from build123d import *

# Parameters (mm, degrees)
BASPROSKE_W                                    = 5
BASPROSKE_H                                    = 22
TOOTHCUT_DEPTH                                 = 32.511902513
TEETHCUTS_COUNT                                = 20
TEETHCUTS_ANGLE                                = 342
BORSKE_R                                       = 3.5
BORE_DEPTH                                     = 50.0000508
FRAISAGE_POUR_VIS_T_TE_FRAIS_E_M21_D           = 2.4
FRAISAGE_POUR_VIS_T_TE_FRAIS_E_M21_CSINK_D     = 4.4
FRAISAGE_POUR_VIS_T_TE_FRAIS_E_M21_CSINK_ANGLE = 90
R_P_TITION_CIRCULAIRE1_COUNT                   = 4


with BuildPart() as part:
    # BasProSke → Base-Revolve (revolve)
    with BuildSketch(Plane(origin=(0, 0, 0), x_dir=(1, 0, 0), z_dir=(0, 1, 0)), mode=Mode.PRIVATE) as base_revolve_sk:
        with Locations((2.5, 11)):
            Rectangle(BASPROSKE_W, BASPROSKE_H)
    revolve(base_revolve_sk.sketch.rotate(Axis((-10, 0, 0), (1, 0, 0)), 180), axis=Axis((-10, 0, 0), (1, 0, 0)))

    # TooCutSke → ToothCut (cut, through all)
    with BuildSketch(Plane(origin=(0, 0, 0), x_dir=(0, 0, -1), z_dir=(1, 0, 0))):
        with BuildLine():
            ThreePointArc((0.986171591, 17.471189616), (0, 17.499), (-0.986171591, 17.471189616))
            ThreePointArc((-0.986171591, 17.471189616), (-1.626916196, 19.798789858), (-2.932850173, 21.829260982))
            ThreePointArc((-2.932850173, 21.829260982), (0, 22.0254), (2.932850173, 21.829260982))
            ThreePointArc((2.932850173, 21.829260982), (1.626916196, 19.798789858), (0.986171591, 17.471189616))
        make_face()
    toothcut = extrude(amount=TOOTHCUT_DEPTH, mode=Mode.SUBTRACT)

    # TeethCuts: ToothCut ×20 about axis
    teethcuts_axis = Axis((-10, 0, 0), (1, 0, 0))
    for i in range(1, TEETHCUTS_COUNT):
        add(toothcut.rotate(teethcuts_axis, i * TEETHCUTS_ANGLE / (TEETHCUTS_COUNT - 1)), mode=Mode.SUBTRACT)

    # BorSke → Bore (cut, symmetric)
    with BuildSketch(Plane(origin=(0, 0, 0), x_dir=(0, 0, -1), z_dir=(1, 0, 0))):
        with Locations(Location((0, 0, 0), (0, 0, 180))):
            Circle(BORSKE_R)
    extrude(amount=BORE_DEPTH, both=True, mode=Mode.SUBTRACT)

    # Fraisage pour vis à tête fraisée M21 (through all)
    with Locations(Plane.ZY):
        with Locations((0, 8)):
            fraisage_pour_vis_t_te_frais_e_m21 = CounterSinkHole(FRAISAGE_POUR_VIS_T_TE_FRAIS_E_M21_D / 2, FRAISAGE_POUR_VIS_T_TE_FRAIS_E_M21_CSINK_D / 2, counter_sink_angle=FRAISAGE_POUR_VIS_T_TE_FRAIS_E_M21_CSINK_ANGLE)

    # Répétition circulaire1: Fraisage pour vis à tête fraisée M21 ×4 about axis
    r_p_tition_circulaire1_axis = Axis((0, 0, 0), (1, 0, 0))
    for i in range(1, R_P_TITION_CIRCULAIRE1_COUNT):
        add(fraisage_pour_vis_t_te_frais_e_m21.rotate(r_p_tition_circulaire1_axis, i * 360 / R_P_TITION_CIRCULAIRE1_COUNT), mode=Mode.SUBTRACT)


solid = part.part
Design review of the part built by this model. Coordinates are the model's own, in mm. A direction names the side the tool comes from. Coordinates: 2 decimals unless noted, no trailing zeros. Write each loop counter-clockwise with the first axis right and the second up, starting at its lowest first coordinate (ties: lowest second). Pieces come first, ordered by that corner, then holes. Notation, with made-up numbers: (87.5, 36) -> (146.5, 36) arc R7 cw to (146.5, 44) -> close; hole circle Ø3 at (85.5, -32). An arc over 180 degrees is marked (long way). Write each question's results on one line, items separated by ' | '. Start each with the question number.
(1) For line 1 along Y through (x, z) = (0.7, -19); line 2 along Y through (x, z) = (4.4, 15.5); line 3 along Z through (x, y) = (2.75, 0.5), list the stretches that pass through material, from the lowest coordinate up. Write a range as from..to.
(2) Tool access review of faces 1 (the face through (2.465, 19.754, 1.607)), 2 (the face through (2.465, -15.037, -12.911)), 3 (the face through (2.46, 14.17, 10.27)): name each direction out of +Z, -Z, +X, -X, +Y, -Y from which nothing blocks a thin tool from reaching the whole face with its end or side.
(3) Clearance check with flat-ended pins moving along their axes: P1, Ø1.5, axis at x = 0.5, y = 4, coming from the +Z side; P2, Ø3, axis at x = 1.5, z = -12.5, coming from the -Y side. State where each tip first meets the part, or that it passes through.
(4) The part is to be moulded in two halves that separate along Z. For faces 4 (the face through (2.46, -7.63, 18.29)), 5 (the face through (2.46, -16.64, 5.42)), 6 (the face through (2.465, -7.678, -18.341)), 7 (the face through (0, 5, 0)), say which applies: pulls with the +Z half, pulls with the -Z half, needs draft (parallel to the pull), parting line crosses it, or undercut.
(5) Take a section at A-A on y = 0. Write out the cut boundary in (x, z).
(6) Take a section at C-C on z = -8. Write out the cut boundary in (x, y), and give its area (3 significant figures).
Results found:
1) line 1: y = -10.49..-8.35, -4.6..-1.32, 1.32..4.6, 8.35..10.49 | line 2: y = -15.61..-13.84, -9.86..9.86, 13.84..15.61 | line 3: z = -17.49..-9.09, -6.91..-3.46, 3.46..6.91, 9.09..17.49
2) face 1: +X, -X, +Y | face 2: +X, -X, -Y | face 3: +X, -X
3) P1: stops at z = 21.76 | P2: stops at y = -15.57
4) face 4: pulls with the +Z half | face 5: undercut | face 6: pulls with the -Z half | face 7: needs draft
5) outline: (0, -17.5) -> (5, -17.5) -> (5, -9.2) -> (1, -9.2) -> (0, -10.2) -> close; (0, -5.8) -> (1, -6.8) -> (5, -6.8) -> (5, -3.5) -> (0, -3.5) -> close; (0, 3.5) -> (5, 3.5) -> (5, 6.8) -> (1, 6.8) -> (0, 5.8) -> close; (0, 10.2) -> (1, 9.2) -> (5, 9.2) -> (5, 17.5) -> (0, 17.5) -> close
6) outline: (0, -18.68) -> (5, -18.68) -> (5, -1.2) -> (1, -1.2) -> (0, -2.2) -> close; (0, 2.2) -> (1, 1.2) -> (5, 1.2) -> (5, 18.68) -> (0, 18.68) -> close | area: 174 mm2
